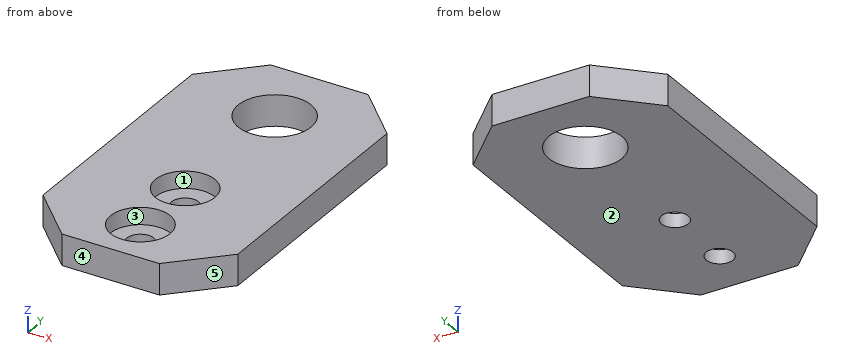
from build123d import *

# Parameters (mm, degrees)
SKETCH1_W                               = 40
SKETCH1_H                               = 70
SKETCH1_R                               = 7.5
BOSS_EXTRUDE1_DEPTH                     = 6.35
CBORE_FOR_M5_HEX_HEAD_BOLT1_D           = 5.5
CBORE_FOR_M5_HEX_HEAD_BOLT1_CBORE_D     = 12.238
CBORE_FOR_M5_HEX_HEAD_BOLT1_CBORE_DEPTH = 3.5
CHAMFER1_SIZE                           = 10


with BuildPart() as part:
    # Sketch1 → Boss-Extrude1 (new body)
    with BuildSketch(Plane.XY):
        Rectangle(SKETCH1_W, SKETCH1_H)
        with Locations((0, 20)):
            Circle(SKETCH1_R, mode=Mode.SUBTRACT)
    extrude(amount=BOSS_EXTRUDE1_DEPTH)

    # CBORE for M5 Hex Head Bolt1 (through all)
    with Locations(Plane.XY.offset(6.35)):
        with Locations((0, -10), (0, -25)):
            CounterBoreHole(CBORE_FOR_M5_HEX_HEAD_BOLT1_D / 2, CBORE_FOR_M5_HEX_HEAD_BOLT1_CBORE_D / 2, CBORE_FOR_M5_HEX_HEAD_BOLT1_CBORE_DEPTH)

    # Chamfer1
    chamfer1_edges = [part.edges().sort_by_distance(p)[0] for p in [
        (-20, 35, 3.175),
        (20, 35, 3.175),
        (20, -35, 3.175),
        (-20, -35, 3.175),
    ]]
    chamfer(chamfer1_edges, length=CHAMFER1_SIZE)


solid = part.part
The listing builds one solid part. Answer for the finished solid, in the listing's coordinates (mm). Face numbers are marked on the shaded views. A direction names the side the tool comes from. Give positions to 0.01 mm unless a question says otherwise; leave off trailing zeros. Order: outer loops, then holes, each group sorted by start corner. A loop starts at its lowest first (then second) coordinate and runs counter-clockwise, first axis right, second up. Notation, with made-up numbers: (32, -5) - (91, -5) arc R35 ccw to (91, 29) - close; hole circle Ø9 at (28, -14.75). An arc over 180 degrees is marked (long way). Answer as CSV lines item,"result".
Q1. Which of the six approach directions +Z, -Z, +X, -X, +Y, -Y give full straight-line access (tool end or side, diameter ignored) to the marked faces 1 and 2?
Answer key:
face 1,"+Z"
face 2,"-Z, +X, -X, +Y, -Y"
Q2. Determine the mould class of the marked faces 3, 4 and 5 for opening direction X: pulls with the +X half, pulls with the -X half, needs draft (parallel to the pull), parting line crosses it, or undercut.
Answer key:
face 3,"undercut"
face 4,"needs draft"
face 5,"pulls with the +X half"
Q3. This flat-tipped pin is pushed along its axis until it touches: pin 1 Ø7 at (x, y) = (0, -25) entering from +Z. Where does it stop, or does it pass through?
Answer key:
pin 1,"stops at z = 2.85"
Q4. A cutting plane is placed at C-C, the plane z = 5.5. Determine the outline of the cut face in (x, y), and give its area (3 significant figures).
Answer key:
outline,"(-20, -25) - (-10, -35) - (10, -35) - (20, -25) - (20, 25) - (10, 35) - (-10, 35) - (-20, 25) - close; hole circle Ø15 at (0, 20); hole circle Ø12.24 at (0, -25); hole circle Ø12.24 at (0, -10)"
area,"2,190 mm^2"
Q5. A cutting plane is placed at A-A, the plane y = 20. Determine the outline of the cut face in (x, z), and give its area (3 significant figures).
Answer key:
outline,"(-20, 0) - (-7.5, 0) - (-7.5, 6.35) - (-20, 6.35) - close; (7.5, 0) - (20, 0) - (20, 6.35) - (7.5, 6.35) - close"
area,"159 mm^2"
Q6. Straight lines are drawn through the part: L1, parallel to Y at x = 0, z = 6; L2, parallel to Y at x = 0, z = 1.95; L3, parallel to X at y = 14, z = 3.75. For each, find the intervals that lie inside material, in ascending order.
Answer key:
L1,"y = -35 to -31.12, -18.88 to -16.12, -3.88 to 12.5, 27.5 to 35"
L2,"y = -35 to -27.75, -22.25 to -12.75, -7.25 to 12.5, 27.5 to 35"
L3,"x = -20 to -4.5, 4.5 to 20"
Q7. A cutting plane is placed at D-D, the plane x = -5. Determine the outline of the cut face in (y, z), and give its area (3 significant figures).
Answer key:
outline,"(-35, 0) - (14.41, 0) - (14.41, 6.35) - (-6.47, 6.35) - (-6.47, 2.85) - (-13.53, 2.85) - (-13.53, 6.35) - (-21.47, 6.35) - (-21.47, 2.85) - (-28.53, 2.85) - (-28.53, 6.35) - (-35, 6.35) - close; (25.59, 0) - (35, 0) - (35, 6.35) - (25.59, 6.35) - close"
area,"324 mm^2"
Q8. A cutting plane is placed at B-B, the plane x = 0. Determine the outline of the cut face in (y, z), and give its area (3 significant figures).
Answer key:
outline,"(-35, 0) - (-27.75, 0) - (-27.75, 2.85) - (-31.12, 2.85) - (-31.12, 6.35) - (-35, 6.35) - close; (-22.25, 0) - (-12.75, 0) - (-12.75, 2.85) - (-16.12, 2.85) - (-16.12, 6.35) - (-18.88, 6.35) - (-18.88, 2.85) - (-22.25, 2.85) - close; (-7.25, 0) - (12.5, 0) - (12.5, 6.35) - (-3.88, 6.35) - (-3.88, 2.85) - (-7.25, 2.85) - close; (27.5, 0) - (35, 0) - (35, 6.35) - (27.5, 6.35) - close"
area,"232 mm^2"
